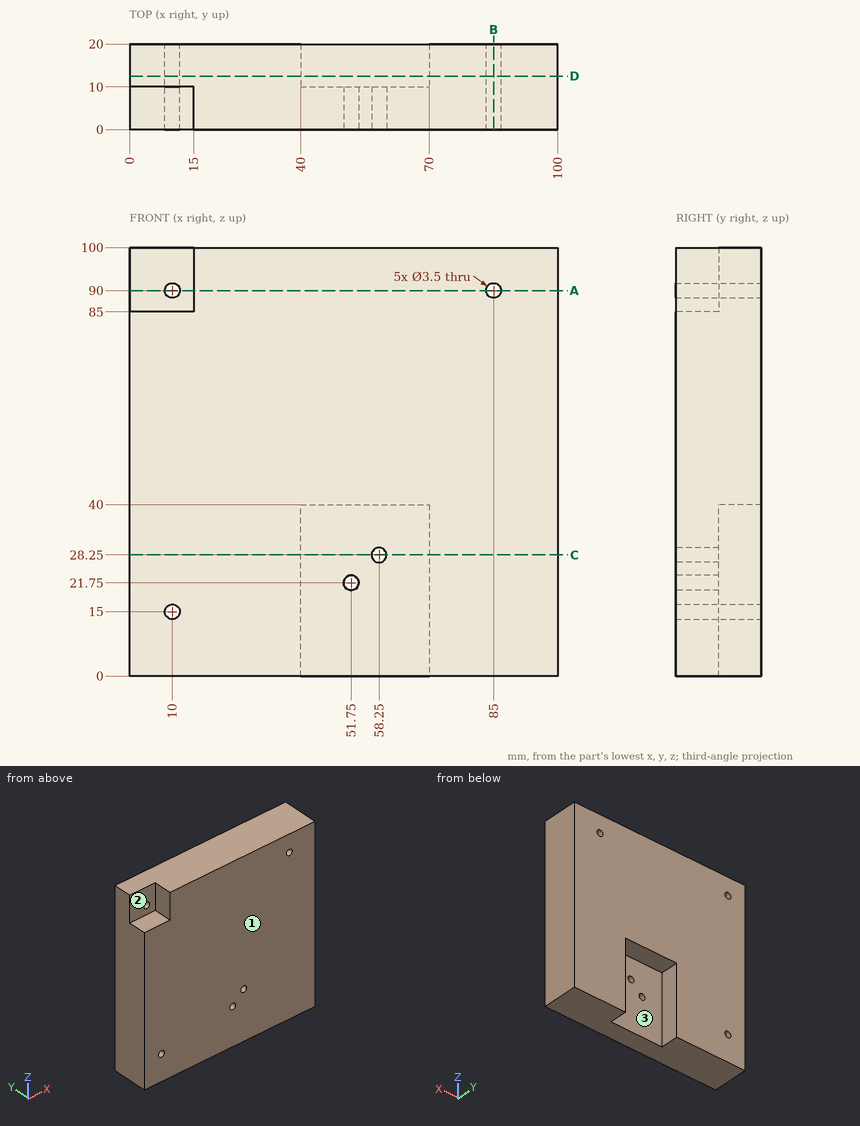
Print and shaded views of the part. All mm, measured from the part's lowest x, y and z. A direction names the side the tool comes from. Coordinates: 2 decimals unless noted, no trailing zeros. Write each loop counter-clockwise with the first axis right and the second up, starting at its lowest first coordinate (ties: lowest second). Pieces come first, ordered by that corner, then holes. Notation, with made-up numbers: M -32.75,1 L -28.75,1 A20 ccw -28.75,37 Z; hole C 43,-0.75 d5. An arc over 180 degrees is marked long. Return JSON: item names as keys, results as strings.
1. Saw through at C-C, the plane z = 28.25. Write the cut outline in (x, y), then the cut area to 4 significant figures.
Determined:
{"outline": "M 0,0 L 56.5,0 L 56.5,10 L 40,10 L 40,20 L 0,20 Z; M 60,0 L 100,0 L 100,20 L 70,20 L 70,10 L 60,10 Z", "area": "1,665 mm²"}
2. Saw through at D-D, the plane y = 12.5. Write the cut outline in (x, z).
Determined:
{"outline": "M 0,0 L 40,0 L 40,40 L 70,40 L 70,0 L 100,0 L 100,100 L 0,100 Z; hole C 10,15 d3.5; hole C 10,90 d3.5; hole C 85,90 d3.5"}
3. Probe L1, parallel to X at y = 10.5, z = 15; L2, parallel to Z at x = 10, y = 14.5; L3, parallel to X at y = 14, z = 90. List the from-to ranges inside material, lowest first.
Determined:
{"L1": "0 to 8.25, 11.75 to 40, 70 to 100", "L2": "0 to 13.25, 16.75 to 88.25, 91.75 to 100", "L3": "0 to 8.25, 11.75 to 83.25, 86.75 to 100"}
4. 3-axis set-ups, long thin cutter, end or side, ignore diameter. For the marked faces 1, 2 and 3: which of +Z, -Z, +X, -X, +Y, -Y reach the whole face in a straight line?
Determined:
{"face 1": "+Z, -Z, +X, -X, -Y", "face 2": "+Z, -X, -Y", "face 3": "-Z, +Y"}
5. Saw through at B-B, the plane x = 85. Write the cut outline in (y, z), then the cut area to 3 significant figures.
Determined:
{"outline": "M 0,0 L 20,0 L 20,88.25 L 0,88.25 Z; M 0,91.75 L 20,91.75 L 20,100 L 0,100 Z", "area": "1,930 mm²"}
6. Saw through at A-A, the plane z = 90. Write the cut outline in (x, y), then the cut area to 4 significant figures.
Determined:
{"outline": "M 0,10 L 8.25,10 L 8.25,20 L 0,20 Z; M 11.75,10 L 15,10 L 15,0 L 83.25,0 L 83.25,20 L 11.75,20 Z; M 86.75,0 L 100,0 L 100,20 L 86.75,20 Z", "area": "1,745 mm²"}
7. Flat gauge pins, fed straight in: pin 1 Ø5 at (x, y) = (8.5, 4) entering from +Z; pin 2 Ø11 at (x, y) = (58.5, 17) entering from -Z; pin 3 Ø9 at (x, z) = (61, 11.5) entering from +Y. Where does each tip first touch, or does it go through?
Determined:
{"pin 1": "z = 85", "pin 2": "z = 40", "pin 3": "y = 10"}
